The figure shows three views and two pictorial views of one solid part (mm, origin at its lowest corner). Answer the questions. Coordinates: 2 decimals unless noted, no trailing zeros. Loops run counter-clockwise (first coordinate to the right, second up) from the corner with the lowest first, then second, coordinate; pieces in that order, holes last. Notation, with made-up numbers: M 10,-37.5 L 47,-37.5 A22 ccw 47,-0.5 Z; hole C 29,59.25 d6. An arc over 180 degrees is marked long. One line per item, written item: value. Start each with the question number.
1. The part is cut by section C-C (z = 0.95). State how many separate pieces and enclosed holes the cut face has, then the cut area to 3 significant figures.
2. The part is cut by section D-D (x = 4). Write down the section's boundary in (y, z) (1 decimal).
3. The part is cut by section A-A (y = 25.75). Write down the section's boundary in (x, z).
4. Consider probe 1 along Y at (x, z) = (41, 0.2); probe 2 along Y at (x, z) = (30, 1.5); probe 3 along Y at (x, z) = (30.5, 0.1). Determine where each line is inside the solid, lowest interval first.
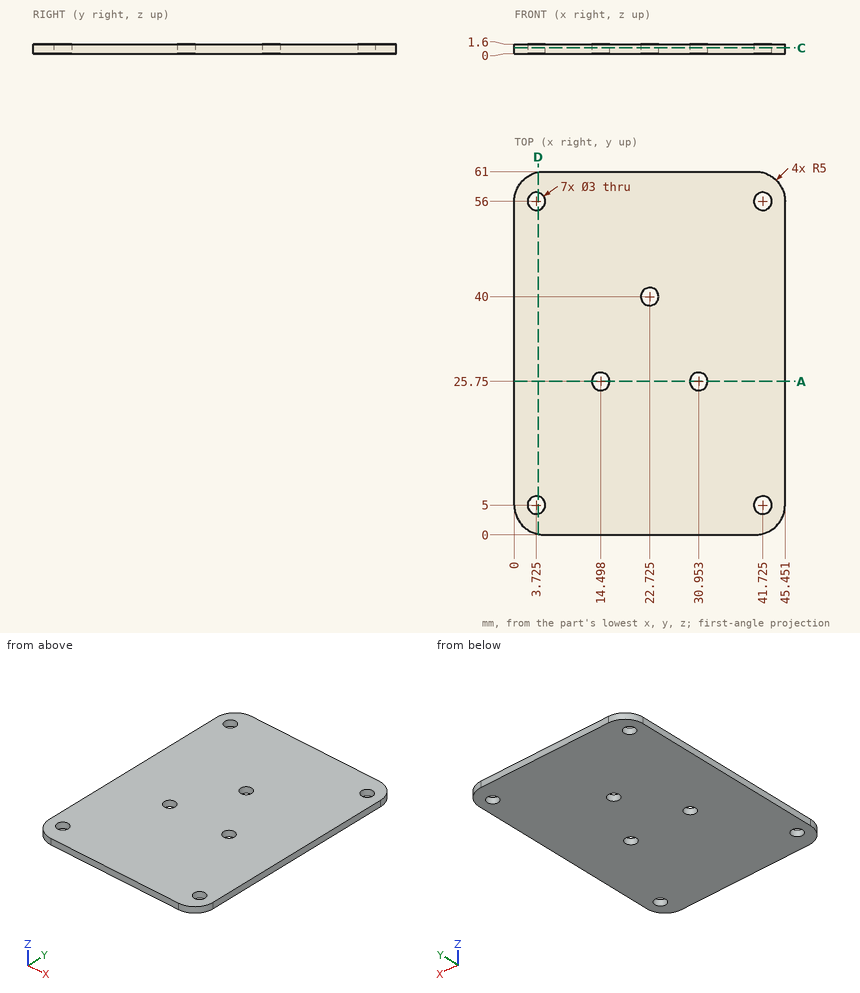
Answer block:
1. separate pieces: 1
1. enclosed holes: 7
1. area: 2,700 mm2
2. outline: M 0.1,0 L 3.5,0 L 3.5,1.6 L 0.1,1.6 Z; M 6.5,0 L 54.5,0 L 54.5,1.6 L 6.5,1.6 Z; M 57.5,0 L 60.9,0 L 60.9,1.6 L 57.5,1.6 Z
3. outline: M 0,0 L 13,0 L 13,1.6 L 0,1.6 Z; M 16,0 L 29.45,0 L 29.45,1.6 L 16,1.6 Z; M 32.45,0 L 45.45,0 L 45.45,1.6 L 32.45,1.6 Z
4. probe 1: y = 0.03 to 3.69, 6.31 to 54.69, 57.31 to 60.97
4. probe 2: y = 0 to 24.59, 26.91 to 61
4. probe 3: y = 0 to 24.32, 27.18 to 61
